The listing builds one solid part. Answer for the finished solid, in the listing's coordinates (mm). Face numbers are marked on the shaded views. Coordinates: 2 decimals unless noted, no trailing zeros. Order: outer loops, then holes, each group sorted by start corner. A loop starts at its lowest first (then second) coordinate and runs counter-clockwise, first axis right, second up. Notation, with made-up numbers: (-12, 60) - (43, 60) arc R27 ccw to (43, 96) - close; hole circle Ø3 at (24, -31.5). An arc over 180 degrees is marked (long way). Use one line per item in the form item = value. Start each with the question number.
Item 1: Section B-B, the plane y = 0 is taken. Write down the section's boundary in (x, z) (3 decimals).
Item 2: Section A-A, the plane x = 0 is taken. Write down the section's boundary in (y, z) (3 decimals), and give its area (3 significant figures).
Item 3: Consider line 1 along Y through (x, z) = (0, 6.75) (3 decimals); line 2 along X through (y, z) = (-6, 1.75); line 3 along X through (y, z) = (11, 8.25). Determine where each line is inside the solid, lowest interval first. Write a range as [from, to].
Item 4: The mould has two halves that part along X. Classify the marked faces 1, 2 and 3: released by +X, released by -X, zero draft, split by the parting line, or undercut.
Item 5: Each of these flat-tipped pins is pushed along its axis until it touches: pin 1 Ø1.8 at (y, z) = (4, 4) entering from -X; pin 2 Ø1.5 at (x, z) = (9, 6) entering from -Y; pin 3 Ø3 at (x, z) = (-0.5, 6) entering from -Y. Where does it stop, or does it pass through?
Item 6: Section D-D, the plane y = -5 is taken. Write down the section's boundary in (x, z), and give its area (3 significant figures).
Item 7: Section C-C, the plane z = 2 is taken. Write down the section's boundary in (x, y) (3 decimals), and give its area (3 significant figures).
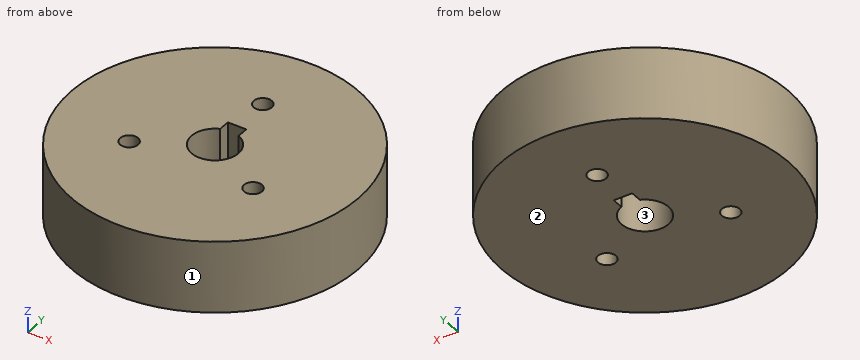
from build123d import *

# Parameters (mm, degrees)
SKETCH1_R               = 20
SKETCH1_R_2             = 1.250479472
SKETCH1_R_3             = 3.275
BOSS_EXTRUDE1_DEPTH     = 10
CUT_EXTRUDE1_DEPTH      = 31
CUT_EXTRUDE1_DEPTH_BACK = 31
SKETCH2_W               = 2.58125
SKETCH2_H               = 4.615625


with BuildPart() as part:
    # Sketch1 → Boss-Extrude1 (new body)
    with BuildSketch(Plane.XY):
        Circle(SKETCH1_R)
        with Locations((0, 10)):
            Circle(SKETCH1_R_2, mode=Mode.SUBTRACT)
        Circle(SKETCH1_R_3, mode=Mode.SUBTRACT)
        with Locations((8.660254038, -5)):
            Circle(SKETCH1_R_2, mode=Mode.SUBTRACT)
        with Locations((-8.660254038, -5)):
            Circle(SKETCH1_R_2, mode=Mode.SUBTRACT)
    extrude(amount=BOSS_EXTRUDE1_DEPTH)

    # Sketch2 → Cut-Extrude1 (cut, two sides: drawn at the far end of the back side and taken through both)
    with BuildSketch(Plane.XY.offset(10).offset(-CUT_EXTRUDE1_DEPTH_BACK)):
        with Locations((0, 2.3078125)):
            Rectangle(SKETCH2_W, SKETCH2_H)
    extrude(amount=CUT_EXTRUDE1_DEPTH + CUT_EXTRUDE1_DEPTH_BACK, mode=Mode.SUBTRACT)


solid = part.part
Response:
q1.outline = (-20, 0) - (-3.275, 0) - (-3.275, 10) - (-20, 10) - close; (3.275, 0) - (20, 0) - (20, 10) - (3.275, 10) - close
q2.outline = (-20, 0) - (-3.275, 0) - (-3.275, 10) - (-20, 10) - close; (4.616, 0) - (8.75, 0) - (8.75, 10) - (4.616, 10) - close; (11.25, 0) - (20, 0) - (20, 10) - (11.25, 10) - close
q2.area = 296 mm2
q3.line_1 = [-20, -3.275], [4.616, 8.75], [11.25, 20]
q3.line_2 = [-19.08, -9.41], [-7.91, 7.91], [9.41, 19.08]
q3.line_3 = [-16.7, -0.75], [0.75, 16.7]
q4.face_1 = split by the parting line
q4.face_2 = zero draft
q4.face_3 = undercut
q5.pin_1 = -19.76
q5.pin_2 = -18.22
q5.pin_3 = -20
q6.outline = (-19.36, 0) - (-9.91, 0) - (-9.91, 10) - (-19.36, 10) - close; (-7.41, 0) - (7.41, 0) - (7.41, 10) - (-7.41, 10) - close; (9.91, 0) - (19.36, 0) - (19.36, 10) - (9.91, 10) - close
q6.area = 337 mm2
q7.outline = circle Ø40 at (0, 0); hole circle Ø2.501 at (-8.66, -5); hole (-1.291, 3.01) arc R3.275 ccw (long way) to (1.291, 3.01) - (1.291, 4.616) - (-1.291, 4.616) - close; hole circle Ø2.501 at (0, 10); hole circle Ø2.501 at (8.66, -5)
q7.area = 1,200 mm2
